from build123d import *

# Parameters (mm, degrees)
F0_R           = 38.1
F0_R_2         = 9.525
F1_DEPTH       = 12.7
F2_R           = 12.333781
F3_DEPTH       = 6.35
F5_D           = 3.175
F5_CBORE_D     = 6.35
F5_CBORE_DEPTH = 6.35
F6_R           = 23.8125
F6_R_2         = 22.225
F7_DEPTH       = 1.905


with BuildPart() as f1:
    # F0 (on Front) → F1 (new body)
    with BuildSketch(Plane.XZ):
        with Locations((0, 1.841663)):
            Circle(F0_R)
        Circle(F0_R_2, mode=Mode.SUBTRACT)
    extrude(amount=F1_DEPTH)

    # F2 (on face) → F3 (cut)
    with BuildSketch(Plane.XZ.offset(12.7)):
        Circle(F2_R)
    extrude(amount=-F3_DEPTH, mode=Mode.SUBTRACT)

    # F5 (through all)
    with Locations(Plane.XZ.offset(12.7)):
        with Locations((0, 31.75), (31.75, 0), (0, -31.75), (-31.75, 0)):
            CounterBoreHole(F5_D / 2, F5_CBORE_D / 2, F5_CBORE_DEPTH)

    # F6 (on face) → F7 (cut)
    with BuildSketch(Plane(origin=(0, 0, 0), x_dir=(-1, 0, 0), z_dir=(0, 1, 0))):
        Circle(F6_R)
        Circle(F6_R_2, mode=Mode.SUBTRACT)
    extrude(amount=-F7_DEPTH, mode=Mode.SUBTRACT)


solid = f1.part
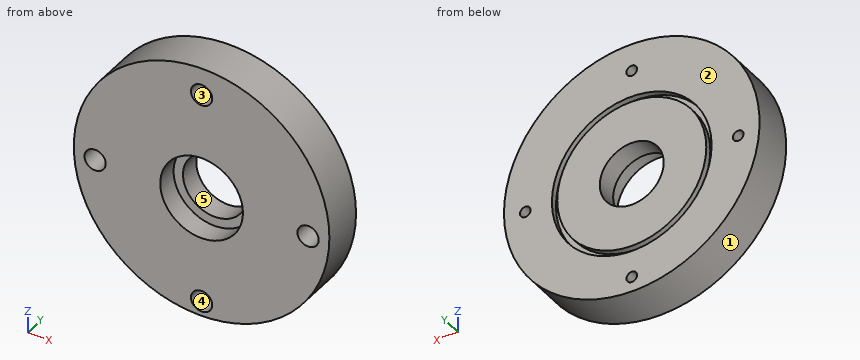
Build history of the part. All positions in model axes, mm. Face numbers are marked on the shaded views. A direction names the side the tool comes from. Round coordinates to 2 decimals unless told otherwise and drop trailing zeros. Write each loop counter-clockwise with the first axis right and the second up, starting at its lowest first coordinate (ties: lowest second). Pieces come first, ordered by that corner, then holes. Notation, with made-up numbers: (70.5, -0.75) -> (120.5, -0.75) arc R28 ccw to (120.5, 38.25) -> close; hole circle Ø8 at (60, 58). An arc over 180 degrees is marked (long way). Use one line per item in the form item = value.
Q1. Band-saw the part on D-D, the plane x = 14.5. Write the cut outline in (y, z) (3 decimals).
Conclusion:
outline = (-12.7, -33.391) -> (0, -33.391) -> (0, -18.889) -> (-1.905, -18.889) -> (-1.905, -16.843) -> (0, -16.843) -> (0, 16.843) -> (-1.905, 16.843) -> (-1.905, 18.889) -> (0, 18.889) -> (0, 37.075) -> (-12.7, 37.075) -> close
Q2. Band-saw the part on C-C, the plane y = -8. Write the cut outline in (x, z) (3 decimals), then the cut area to 3 significant figures.
Conclusion:
outline = circle Ø76.2 at (0, 1.842); hole circle Ø6.35 at (-31.75, 0); hole circle Ø24.668 at (0, 0); hole circle Ø6.35 at (0, -31.75); hole circle Ø6.35 at (0, 31.75); hole circle Ø6.35 at (31.75, 0)
area = 3,960 mm²
Q3. Two-plate mould, pull along X, no slides. Class the marked faces 1, 2 and 3: released by +X, released by -X, zero draft, split by the parting line, or undercut.
Conclusion:
face_1 = split by the parting line
face_2 = zero draft
face_3 = undercut
Q4. Drop flat-ended pins along their axis: P1, Ø1.5, axis at x = -0.5, y = -8, coming from the -Z side; P2, Ø1.9, axis at x = 33.5, z = 0, coming from the -Y side; P3, Ø4, axis at x = 6, y = -11.5, coming from the -Z side. Give the stop position or say it passes through.
Conclusion:
P1 = -36.26
P2 = -6.35
P3 = -36.05
Q5. Drill centre lines: L1, parallel to Z at x = 0, y = -0.35 (1 decimal); L2, parallel to Z at x = 0, y = -2.5 (1 decimal); L3, parallel to X at y = -6.5, z = -1. Where is each one in solid material? Low to high.
Conclusion:
L1 = -36.3 to -33.3, -30.2 to -23.8, -22.2 to -9.5, 9.5 to 22.2, 23.8 to 30.2, 33.3 to 39.9
L2 = -36.3 to -33.3, -30.2 to -9.5, 9.5 to 30.2, 33.3 to 39.9
L3 = -37.99 to -34.76, -28.74 to -12.29, 12.29 to 28.74, 34.76 to 37.99
Q6. Band-saw the part on A-A, the plane z = 7. Write the cut outline in (x, y) (3 decimals).
Conclusion:
outline = (-37.749, -12.7) -> (-10.155, -12.7) -> (-10.155, -6.35) -> (-6.46, -6.35) -> (-6.46, 0) -> (-21.094, 0) -> (-21.094, -1.905) -> (-22.76, -1.905) -> (-22.76, 0) -> (-37.749, 0) -> close; (6.46, -6.35) -> (10.155, -6.35) -> (10.155, -12.7) -> (37.749, -12.7) -> (37.749, 0) -> (22.76, 0) -> (22.76, -1.905) -> (21.094, -1.905) -> (21.094, 0) -> (6.46, 0) -> close
Q7. Tool access for the marked faces 4 and 5: list every direction of +Z, -Z, +X, -X, +Y, -Y with a clear straight run to the whole face (end or side of a thin tool).
Conclusion:
face_4 = -Y
face_5 = +Y, -Y
